Could you check a few things on this model? Use its own coordinates, in mm. A direction names the side the tool comes from. Round coordinates to 2 decimals unless told otherwise and drop trailing zeros. Write each loop counter-clockwise with the first axis right and the second up, starting at its lowest first coordinate (ties: lowest second). Pieces come first, ordered by that corner, then holes.
```python
from build123d import *


with BuildPart() as part:
    # Sketch1 → Revolve1 (revolve)
    with BuildSketch(Plane.XY):
        with BuildLine():
            Line((-2.5, -47.669872981), (-2.5, -25.7))
            Line((-2.5, -25.7), (-6.75, -25.7))
            Line((-6.75, -25.7), (-7.75, -17.2))
            Line((-7.75, -17.2), (-16, -17.2))
            Line((-16, -17.2), (-17.75, 0))
            Line((-17.75, 0), (-16, 17.2))
            Line((-16, 17.2), (-10.75, 17.2))
            Line((-10.75, 17.2), (-10.25, 24.2))
            Line((-10.25, 24.2), (-3.35, 24.2))
            Line((-3.35, 24.2), (-3.35, 27.2))
            ThreePointArc((-3.35, 27.2), (-1.699733397, 26.767694664), (0, 26.622181276))
            Line((0, 26.622181276), (0, -57))
            ThreePointArc((0, -57), (-4.829629131, -53.294095226), (-2.5, -47.669872981))
        make_face()
    revolve(axis=Axis((0, -52, 0), (0, 1, 0)))


solid = part.part
```
Q1. I'm going to push flat-ended pins straight in: pin 1 Ø5 at (x, y) = (-11, 7.5) entering from +Z; pin 2 Ø4 at (x, z) = (3.5, 0.5) entering from -Y; pin 3 Ø12 at (y, z) = (8, -1) entering from -X. Where does each tip first touch, or does it pass through?
Q2. Imagine slicing it at D-D, the plane y = 21. Write out the boundary of the cut face in (x, z), then the cut area to 3 significant figures.
Q3. Imagine slicing it at C-C, the plane y = -36. Write out the boundary of the cut face in (x, z), then the cut area to 3 significant figures.
Q4. We'd pull the mould along Y, two halves only. Please class faces 4 (the conical face through (-3.3, -22.33, -6.34)), 5 (the flat face through (-10.4, 17.2, -3.3)), 6 (the cylindrical face through (0.54, -36.53, -2.44)): pulls with the +Y half, pulls with the -Y half, needs draft (parallel to the pull), parting line crosses it, or undercut.
Q5. Imagine slicing it at A-A, the plane z = 0. Write out the boundary of the cut face in (x, y).
Q6. Imagine slicing it at B-B, the plane x = 0. Write out the boundary of the cut face in (y, z), then the cut area to 3 significant figures.
Q7. If I drill on L1, parallel to Y at x = 4, z = 3.5; L2, parallel to Y at x = 4.5, z = -14.5; L3, parallel to Y at x = 2, z = 2.5, over which ranges is the centre line in solid material (lowest first)?
Q8. On a 3-axis mill with a long thin cutter (end or side, diameter ignored), from which of +Z, -Z, +X, -X, +Y, -Y can I reach the whole of each face in a straight line? I mean faces 1 (the flat face through (7, -17.2, 4)), 2 (the cylindrical face through (3.347, 25.721, 0.147)), 3 (the flat face through (3, -25.7, 0)). Say none if no direction works.
Results found:
1. pin 1: stops at z = 14.74
1. pin 2: stops at y = -56.76
1. pin 3: stops at x = -17.54
2. outline: circle Ø20.96 at (0, 0)
2. area: 345 mm2
3. outline: circle Ø5 at (0, 0)
3. area: 19.6 mm2
4. face 4: pulls with the -Y half
4. face 5: pulls with the +Y half
4. face 6: undercut
5. outline: (-17.75, 0) - (-16, -17.2) - (-7.75, -17.2) - (-6.75, -25.7) - (-2.5, -25.7) - (-2.5, -47.67) arc R5 ccw (long way) to (2.5, -47.67) - (2.5, -25.7) - (6.75, -25.7) - (7.75, -17.2) - (16, -17.2) - (17.75, 0) - (16, 17.2) - (10.75, 17.2) - (10.25, 24.2) - (3.35, 24.2) - (3.35, 27.2) arc R10 cw to (-3.35, 27.2) - (-3.35, 24.2) - (-10.25, 24.2) - (-10.75, 17.2) - (-16, 17.2) - close
6. outline: (-47.67, -2.5) - (-25.7, -2.5) - (-25.7, -6.75) - (-17.2, -7.75) - (-17.2, -16) - (0, -17.75) - (17.2, -16) - (17.2, -10.75) - (24.2, -10.25) - (24.2, -3.35) - (27.2, -3.35) arc R10 cw to (27.2, 3.35) - (24.2, 3.35) - (24.2, 10.25) - (17.2, 10.75) - (17.2, 16) - (0, 17.75) - (-17.2, 16) - (-17.2, 7.75) - (-25.7, 6.75) - (-25.7, 2.5) - (-47.67, 2.5) arc R5 ccw (long way) to start
6. area: 1,630 mm2
7. L1: y = -25.7 to 24.2
7. L2: y = -17.2 to 17.2
7. L3: y = -55.84 to -48.16, -25.7 to 27.15
8. face 1: -Y
8. face 2: +Y
8. face 3: none
